```python
from build123d import *

# Parameters (mm, degrees)
SKETCH1_R           = 1.5
SKETCH1_R_2         = 70
BOSS_EXTRUDE2_DEPTH = 6.35
FILLET1_R           = 30
CIRPATTERN1_DEPTH   = 6.35


# Read off the part's stored shape, not the designer's step: CirPattern1
with BuildPart() as part:
    # Sketch1 → Boss-Extrude2 (new body)
    with BuildSketch(Plane.XY):
        with BuildLine():
            ThreePointArc((80, -140), (128.664709099, -74.284604433), (161.24355653, 0.717967697))
            Line((161.24355653, 0.717967697), (81.24355653, 139.282032303))
            ThreePointArc((81.24355653, 139.282032303), (0, 148.569208867), (-81.24355653, 139.282032303))
            Line((-81.24355653, 139.282032303), (-161.24355653, 0.717967697))
            ThreePointArc((-161.24355653, 0.717967697), (-128.664709099, -74.284604433), (-80, -140))
            Line((-80, -140), (80, -140))
        make_face()
        with Locations((85.333302492, 112.198384506)):
            Circle(SKETCH1_R, mode=Mode.SUBTRACT)
        with Locations((-85.333302492, 112.198384506)):
            Circle(SKETCH1_R, mode=Mode.SUBTRACT)
        with Locations((-69.5, -130)):
            Circle(SKETCH1_R, mode=Mode.SUBTRACT)
        with Locations((-54.5, -130)):
            Circle(SKETCH1_R, mode=Mode.SUBTRACT)
        with Locations((-69.5, -74)):
            Circle(SKETCH1_R, mode=Mode.SUBTRACT)
        with Locations((-54.5, -74)):
            Circle(SKETCH1_R, mode=Mode.SUBTRACT)
        with Locations((-98.83587988, -23.188765563)):
            Circle(SKETCH1_R, mode=Mode.SUBTRACT)
        with Locations((54.5, -130)):
            Circle(SKETCH1_R, mode=Mode.SUBTRACT)
        with Locations((69.5, -130)):
            Circle(SKETCH1_R, mode=Mode.SUBTRACT)
        with Locations((54.5, -74)):
            Circle(SKETCH1_R, mode=Mode.SUBTRACT)
        with Locations((69.5, -74)):
            Circle(SKETCH1_R, mode=Mode.SUBTRACT)
        with Locations((98.83587988, -23.188765563)):
            Circle(SKETCH1_R, mode=Mode.SUBTRACT)
        with Locations((-147.333302492, 4.811234437)):
            Circle(SKETCH1_R, mode=Mode.SUBTRACT)
        with Locations((-91.33587988, -10.198384506)):
            Circle(SKETCH1_R, mode=Mode.SUBTRACT)
        with Locations((-139.833302492, 17.801615494)):
            Circle(SKETCH1_R, mode=Mode.SUBTRACT)
        Circle(SKETCH1_R_2, mode=Mode.SUBTRACT)
        with Locations((-36.83587988, 84.198384506)):
            Circle(SKETCH1_R, mode=Mode.SUBTRACT)
        with Locations((-29.33587988, 97.188765563)):
            Circle(SKETCH1_R, mode=Mode.SUBTRACT)
        with Locations((91.33587988, -10.198384506)):
            Circle(SKETCH1_R, mode=Mode.SUBTRACT)
        with Locations((147.333302492, 4.811234437)):
            Circle(SKETCH1_R, mode=Mode.SUBTRACT)
        with Locations((139.833302492, 17.801615494)):
            Circle(SKETCH1_R, mode=Mode.SUBTRACT)
        with Locations((36.83587988, 84.198384506)):
            Circle(SKETCH1_R, mode=Mode.SUBTRACT)
        with Locations((29.33587988, 97.188765563)):
            Circle(SKETCH1_R, mode=Mode.SUBTRACT)
        with Locations((77.833302492, 125.188765563)):
            Circle(SKETCH1_R, mode=Mode.SUBTRACT)
        with Locations((-77.833302492, 125.188765563)):
            Circle(SKETCH1_R, mode=Mode.SUBTRACT)
    extrude(amount=BOSS_EXTRUDE2_DEPTH)

    # Fillet1
    fillet1_edges = [part.edges().sort_by_distance(p)[0] for p in [
        (-161.24355653, 0.717967697, 3.175),
        (-81.24355653, 139.282032303, 3.175),
    ]]
    fillet(fillet1_edges, radius=FILLET1_R)

    # CirPattern1 outline → CirPattern1 (cut)
    with BuildSketch(Plane.XY):
        with BuildLine():
            ThreePointArc((81.24355653, 139.282032303), (74.425715453, 140.791884002), (67.57987135, 142.169210265))
            ThreePointArc((67.57987135, 142.169210265), (79.330889418, 137.153364411), (87.928977518, 127.702543481))
            Line((87.928977518, 127.702543481), (81.24355653, 139.282032303))
        make_face()
        with BuildLine():
            Line((-80, -140), (-66.629158024, -140))
            ThreePointArc((-66.629158024, -140), (-79.112853086, -137.279247746), (-89.33221205, -129.610490506))
            ThreePointArc((-89.33221205, -129.610490506), (-84.716490466, -134.850502278), (-80, -140))
        make_face()
        with BuildLine():
            ThreePointArc((80, -140), (84.716490466, -134.850502278), (89.33221205, -129.610490506))
            ThreePointArc((89.33221205, -129.610490506), (79.112853086, -137.279247746), (66.629158024, -140))
            Line((66.629158024, -140), (80, -140))
        make_face()
        with BuildLine():
            Line((161.24355653, 0.717967697), (154.558135542, 12.297456519))
            ThreePointArc((154.558135542, 12.297456519), (158.443742503, 0.125883335), (156.9120834, -12.558719758))
            ThreePointArc((156.9120834, -12.558719758), (159.142205919, -5.941381724), (161.24355653, 0.717967697))
        make_face()
    extrude(amount=CIRPATTERN1_DEPTH, mode=Mode.SUBTRACT)


solid = part.part
```
Can you work these out from the model? Positions are in its coordinate system, mm. Round coordinates to 2 decimals unless told otherwise and drop trailing zeros. Order: outer loops, then holes, each group sorted by start corner. A loop starts at its lowest first (then second) coordinate and runs counter-clockwise, first axis right, second up.
(1) If I drill on L1, parallel to X at y = -73.5, z = 4.5; L2, parallel to Y at x = -30, z = 6; L3, parallel to X at y = -74, z = 4.5, over which ranges is the centre line in solid material (lowest first)?
Results are:
L1: x = -129.12 to -70.91, -68.09 to -55.91, -53.09 to 53.09, 55.91 to 68.09, 70.91 to 129.12
L2: y = -140 to -63.25, 63.25 to 95.84, 98.53 to 147.32
L3: x = -128.83 to -71, -68 to -56, -53 to 53, 56 to 68, 71 to 128.83
(2) If we section it at A-A (y = 48.5): Please give me the cut outline in (x, z).
Results are:
outline: (-133.66, 0) - (-50.48, 0) - (-50.48, 6.35) - (-133.66, 6.35) - close; (50.48, 0) - (133.66, 0) - (133.66, 6.35) - (50.48, 6.35) - close
(3) If we section it at D-D (x = -104): Please give me the cut outline in (y, z).
Results are:
outline: (-111.47, 0) - (99.87, 0) - (99.87, 6.35) - (-111.47, 6.35) - close
(4) If we section it at C-C (z = 1): Count the separate pieces of the cut face and the enclosed holes in it, plus the area to 3 significant figures.
Results are:
separate pieces: 1
enclosed holes: 25
area: 54,900 mm2
(5) If we section it at B-B (x = 43): Please give me the cut outline in (y, z), plus the area to 3 significant figures.
Results are:
outline: (-140, 0) - (-55.24, 0) - (-55.24, 6.35) - (-140, 6.35) - close; (55.24, 0) - (145.99, 0) - (145.99, 6.35) - (55.24, 6.35) - close
area: 1,110 mm2
(6) We'd pull the mould along Y, two halves only. Please class faces 1 (the face through (-55.55, -42.594, 3.131)), 2 (the face through (-79.18, 137.26, 3.22)), 3 (the face through (-2.2, 70.4, 6.35)): +Y half, -Y half, draft (parallel to the pull), parting line (faces both ways), or undercut.
Results are:
face 1: undercut
face 2: +Y half
face 3: draft
(7) I'm going to push flat-ended pins straight in: pin 1 (2 mm diameter, centred on y = -38.5, z = 2, fed in from -X); pin 2 (5 mm diameter, centred on x = -85.33, y = 112.2, fed in from +Z); pin 3 (3 mm diameter, centred on y = -82, z = 3.5, fed in from +X); pin 4 (3 mm diameter, centred on y = -30.5, z = 0.5, fed in from +X). Where does each tip first touch, or does it pass through?
Results are:
pin 1: stops at x = -147.18
pin 2: stops at z = 6.35
pin 3: stops at x = 124.99
pin 4: stops at x = 150.74
